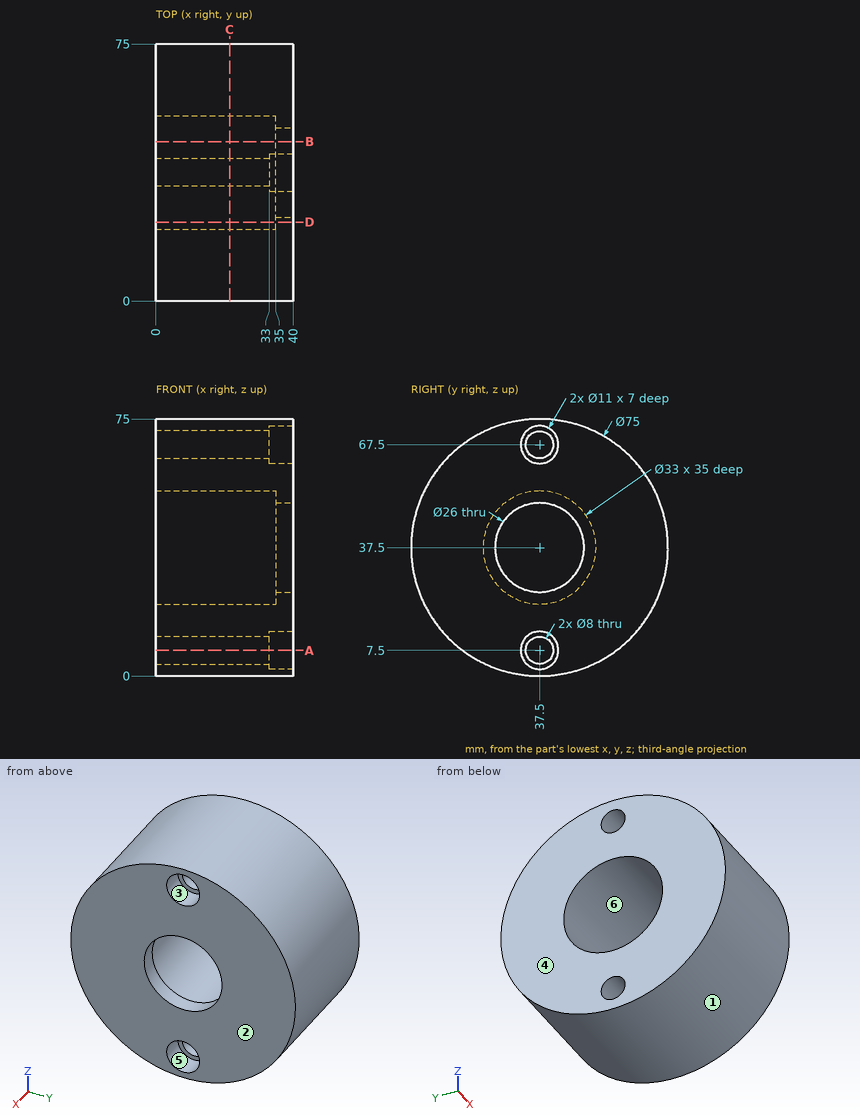
Input: dimensioned drawing with shaded views. Units: mm. Origin: part minimum x, y, z. A direction names the side the tool comes from. Coordinates: 2 decimals unless noted, no trailing zeros. Loops run counter-clockwise (first coordinate to the right, second up) from the corner with the lowest first, then second, coordinate; pieces in that order, holes last. Notation, with made-up numbers: M 67.5,6.5 L 71.5,6.5 A30 cw 71.5,42.5 Z; hole C 20,87.25 d2. An arc over 180 degrees is marked long. Use a Markdown table: item, result. Add a question column.
Q1. Access query for the marked faces 4, 5 and 6. Directions: +Z, -Z, +X, -X, +Y, -Y. A direction counts if a zero-diameter tool reaches every point of the face in a straight line with its end or side. Return the directions, or none.
Q2. Section query D-D, the plane y = 23. Return loops of the section in (x, z), and give its area (3 significant figures).
Q3. Section query A-A, the plane z = 7.5. Return loops of the section in (x, y), and give its area (3 significant figures).
Q4. Section query C-C, the plane x = 21.5. Return loops of the section in (y, z), and give its area (3 significant figures).
Q5. First-contact query: pin 1 (6 mm diameter, centred on x = 19, z = 58.5, fed in from -Y); pin 2 (9 mm diameter, centred on y = 35.5, z = 65.5, fed in from +X); pin 3 (2 mm diameter, centred on x = 4, z = 59.5, fed in from -Y); pin 4 (5 mm diameter, centred on x = 26, z = 51.5, fed in from +Y). Flat tips, straight axial feed; report the tip coordinate or a pass-through.
Q6. Section query B-B, the plane y = 46.5. Return loops of the section in (x, z), and give its area (3 significant figures).
Q7. Draft query along Y for the marked faces 1, 2 and 3. Return one class per face: pulls with the +Y half, pulls with the -Y half, needs draft (parallel to the pull), parting line crosses it, or undercut.
Q8. Material intervals for L1, parallel to Y at x = 18, z = 37; L2, parallel to Z at x = 21, y = 37; L3, parallel to Z at x = 20.5, y = 34, sorted ascending.
Result:
| question | item | result |
|---|---|---|
| 1 | face 4 | +Z, -Z, -X, +Y, -Y |
| 1 | face 5 | +X |
| 1 | face 6 | -X |
| 2 | outline | M 0,2.92 L 40,2.92 L 40,72.08 L 0,72.08 L 0,45.37 L 35,45.37 L 35,29.63 L 0,29.63 Z |
| 2 | area | 2,220 mm2 |
| 3 | outline | M 0,15 L 40,15 L 40,32 L 33,32 L 33,33.5 L 0,33.5 Z; M 0,41.5 L 33,41.5 L 33,43 L 40,43 L 40,60 L 0,60 Z |
| 3 | area | 1,460 mm2 |
| 4 | outline | C 37.5,37.5 d75; hole C 37.5,37.5 d33; hole C 37.5,7.5 d8; hole C 37.5,67.5 d8 |
| 4 | area | 3,460 mm2 |
| 5 | pin 1 | stops at y = 4.6 |
| 5 | pin 2 | stops at x = 40 |
| 5 | pin 3 | stops at y = 6.43 |
| 5 | pin 4 | stops at y = 73.19 |
| 6 | outline | M 0,1.1 L 40,1.1 L 40,28.12 L 35,28.12 L 35,23.67 L 0,23.67 Z; M 0,51.33 L 35,51.33 L 35,46.88 L 40,46.88 L 40,73.9 L 0,73.9 Z |
| 6 | area | 1,850 mm2 |
| 7 | face 1 | parting line crosses it |
| 7 | face 2 | needs draft |
| 7 | face 3 | undercut |
| 8 | L1 | y = 0 to 21.01, 53.99 to 75 |
| 8 | L2 | z = 0 to 3.53, 11.47 to 21.01, 53.99 to 63.53, 71.47 to 75 |
| 8 | L3 | z = 0.16 to 5.56, 9.44 to 21.38, 53.62 to 65.56, 69.44 to 74.84 |
